Can you work these out from the model? Positions are in its coordinate system, mm. Face numbers are marked on the shaded views. A direction names the side the tool comes from. Give positions to 0.01 mm unless a question says otherwise; leave off trailing zeros. Order: outer loops, then holes, each group sorted by start corner. A loop starts at its lowest first (then second) coordinate and runs counter-clockwise, first axis right, second up. Notation, with made-up numbers: M -38.75,-9.75 L -21.75,-9.75 A32 cw -21.75,26.25 Z; hole C 76.25,0.25 d1. An arc over 180 degrees is marked long. Answer as a JSON object with one key per item and string values.
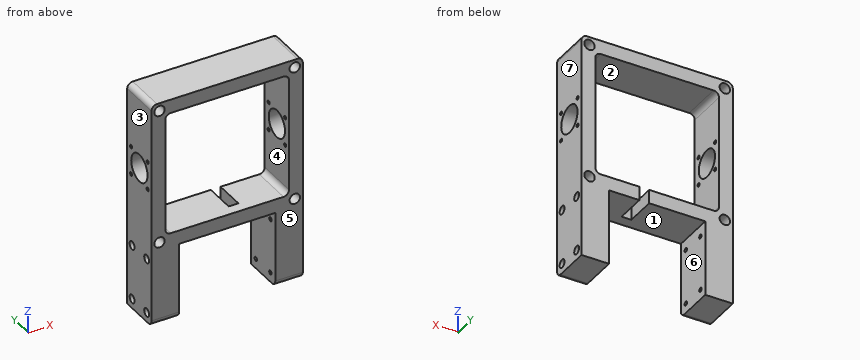
```python
from build123d import *

# Parameters (mm, degrees)
SKETCH1_W           = 25.4
SKETCH1_H           = 69.85
SKETCH1_R           = 4.826
SKETCH1_W_2         = 114.3
SKETCH1_H_2         = 114.3
BOSS_EXTRUDE2_DEPTH = 38.1
CUT_EXTRUDE1_REACH  = 203.206
SKETCH5_R           = 1.63195
SKETCH5_R_2         = 12.75
SKETCH7_W           = 12.7
SKETCH7_H           = 27.94
CUT_EXTRUDE2_DEPTH  = 4.5
CUT_EXTRUDE3_REACH  = 203.206
SKETCH10_R          = 1.905
SKETCH10_3_R        = 3.81
SKETCH10_3_R_2      = 1.905
CUT_EXTRUDE4_DEPTH  = 15.24
CUT_EXTRUDE5_START  = -15.24
SKETCH11_R          = 3.81
CUT_EXTRUDE5_DEPTH  = 15.24
FILLET10_R          = 5.08
FILLET11_R          = 5.08
FILLET12_R          = 5.08
FILLET13_R          = 5.08
FILLET14_R          = 5.08
FILLET15_R          = 5.08
FILLET16_R          = 5.08


with BuildPart() as part:
    # Sketch1 → Boss-Extrude2 (new body)
    # profile 1 of 3: a face of its own
    with BuildSketch(Plane(origin=(0, 0, 0), x_dir=(1, 0, 0), z_dir=(0, 1, 0))):
        with Locations((-57.15, 104.775)):
            Rectangle(SKETCH1_W, SKETCH1_H)
    # profile 2 of 3: a face of its own
    with BuildSketch(Plane(origin=(0, 0, 0), x_dir=(1, 0, 0), z_dir=(0, 1, 0))):
        Polygon((-44.45, 69.85), (-69.85, 69.85), (-69.85, -69.85), (69.85, -69.85), (69.85, 69.85), (44.45, 69.85), (-31.75, 69.85), align=None)
        with Locations(Location((-62.484, -62.484, 0), (0, 0, 90))):
            Circle(SKETCH1_R, mode=Mode.SUBTRACT)
        Rectangle(SKETCH1_W_2, SKETCH1_H_2, mode=Mode.SUBTRACT)
        with Locations(Location((62.484, -62.484, 0), (0, 0, 90))):
            Circle(SKETCH1_R, mode=Mode.SUBTRACT)
        with Locations(Location((-62.484, 62.484, 0), (0, 0, 90))):
            Circle(SKETCH1_R, mode=Mode.SUBTRACT)
        with Locations(Location((62.484, 62.484, 0), (0, 0, 90))):
            Circle(SKETCH1_R, mode=Mode.SUBTRACT)
    # profile 3 of 3: a face of its own
    with BuildSketch(Plane(origin=(0, 0, 0), x_dir=(1, 0, 0), z_dir=(0, 1, 0))):
        with Locations((57.15, 104.775)):
            Rectangle(SKETCH1_W, SKETCH1_H)
    extrude(amount=BOSS_EXTRUDE2_DEPTH)

    # Cut-Extrude1: up to this face of the body (flat: up to its plane)
    cut_extrude1_end = Plane(part.part.faces().sort_by_distance((-69.85, 19.05, -34.925))[0])
    # Sketch5 → Cut-Extrude1 (cut, up to the picked face)
    with BuildSketch(Plane(origin=(69.85, 0, 0), x_dir=(0, 0, -1), z_dir=(1, 0, 0)), mode=Mode.PRIVATE) as cut_extrude1_sk1:
        with Locations((-13, 32.05)):
            Circle(SKETCH5_R)
    cut_extrude1_tool1 = split(extrude(cut_extrude1_sk1.sketch, amount=-CUT_EXTRUDE1_REACH, mode=Mode.PRIVATE), bisect_by=cut_extrude1_end, keep=Keep.BOTH, mode=Mode.PRIVATE)
    # Sketch5 → Cut-Extrude1 (cut, up to the picked face)
    with BuildSketch(Plane(origin=(69.85, 0, 0), x_dir=(0, 0, -1), z_dir=(1, 0, 0)), mode=Mode.PRIVATE) as cut_extrude1_sk2:
        with Locations((13, 6.05)):
            Circle(SKETCH5_R)
    cut_extrude1_tool2 = split(extrude(cut_extrude1_sk2.sketch, amount=-CUT_EXTRUDE1_REACH, mode=Mode.PRIVATE), bisect_by=cut_extrude1_end, keep=Keep.BOTH, mode=Mode.PRIVATE)
    # Sketch5 → Cut-Extrude1 (cut, up to the picked face)
    with BuildSketch(Plane(origin=(69.85, 0, 0), x_dir=(0, 0, -1), z_dir=(1, 0, 0)), mode=Mode.PRIVATE) as cut_extrude1_sk3:
        with Locations((-13, 6.05)):
            Circle(SKETCH5_R)
    cut_extrude1_tool3 = split(extrude(cut_extrude1_sk3.sketch, amount=-CUT_EXTRUDE1_REACH, mode=Mode.PRIVATE), bisect_by=cut_extrude1_end, keep=Keep.BOTH, mode=Mode.PRIVATE)
    # Sketch5 → Cut-Extrude1 (cut, up to the picked face)
    with BuildSketch(Plane(origin=(69.85, 0, 0), x_dir=(0, 0, -1), z_dir=(1, 0, 0)), mode=Mode.PRIVATE) as cut_extrude1_sk4:
        with Locations((13, 32.05)):
            Circle(SKETCH5_R)
    cut_extrude1_tool4 = split(extrude(cut_extrude1_sk4.sketch, amount=-CUT_EXTRUDE1_REACH, mode=Mode.PRIVATE), bisect_by=cut_extrude1_end, keep=Keep.BOTH, mode=Mode.PRIVATE)
    # Sketch5 → Cut-Extrude1 (cut, up to the picked face)
    with BuildSketch(Plane(origin=(69.85, 0, 0), x_dir=(0, 0, -1), z_dir=(1, 0, 0)), mode=Mode.PRIVATE) as cut_extrude1_sk5:
        with Locations((0, 19.05)):
            Circle(SKETCH5_R_2)
    cut_extrude1_tool5 = split(extrude(cut_extrude1_sk5.sketch, amount=-CUT_EXTRUDE1_REACH, mode=Mode.PRIVATE), bisect_by=cut_extrude1_end, keep=Keep.BOTH, mode=Mode.PRIVATE)
    add(cut_extrude1_tool1.solids().sort_by(Axis((69.85, 32.05, 13), (-1, 0, 0)))[0], mode=Mode.SUBTRACT)
    add(cut_extrude1_tool2.solids().sort_by(Axis((69.85, 6.05, -13), (-1, 0, 0)))[0], mode=Mode.SUBTRACT)
    add(cut_extrude1_tool3.solids().sort_by(Axis((69.85, 6.05, 13), (-1, 0, 0)))[0], mode=Mode.SUBTRACT)
    add(cut_extrude1_tool4.solids().sort_by(Axis((69.85, 32.05, -13), (-1, 0, 0)))[0], mode=Mode.SUBTRACT)
    add(cut_extrude1_tool5.solids().sort_by(Axis((69.85, 19.05, 0), (-1, 0, 0)))[0], mode=Mode.SUBTRACT)

    # Sketch7 → Cut-Extrude2 (cut, symmetric)
    with BuildSketch(Plane.ZY.offset(-11.879999989)):
        with Locations((-63.5, 24.13)):
            Rectangle(SKETCH7_W, SKETCH7_H)
    extrude(amount=CUT_EXTRUDE2_DEPTH, both=True, mode=Mode.SUBTRACT)

    # Cut-Extrude3: up to this face of the body (flat: up to its plane)
    cut_extrude3_end = Plane(part.part.faces().sort_by_distance((-69.85, 19.05, -37.47957558))[0])
    # Sketch10 → Cut-Extrude3 (cut, up to the picked face)
    with BuildSketch(Plane(origin=(69.85, 0, 0), x_dir=(0, 0, -1), z_dir=(1, 0, 0)), mode=Mode.PRIVATE) as cut_extrude3_sk1:
        with Locations((80.01, 30.48)):
            Circle(SKETCH10_R)
    cut_extrude3_tool1 = split(extrude(cut_extrude3_sk1.sketch, amount=-CUT_EXTRUDE3_REACH, mode=Mode.PRIVATE), bisect_by=cut_extrude3_end, keep=Keep.BOTH, mode=Mode.PRIVATE)
    # Sketch10 → Cut-Extrude3 (cut, up to the picked face)
    with BuildSketch(Plane(origin=(69.85, 0, 0), x_dir=(0, 0, -1), z_dir=(1, 0, 0)), mode=Mode.PRIVATE) as cut_extrude3_sk2:
        with Locations((80.01, 7.62)):
            Circle(SKETCH10_R)
    cut_extrude3_tool2 = split(extrude(cut_extrude3_sk2.sketch, amount=-CUT_EXTRUDE3_REACH, mode=Mode.PRIVATE), bisect_by=cut_extrude3_end, keep=Keep.BOTH, mode=Mode.PRIVATE)
    # Sketch10 → Cut-Extrude3 (cut, up to the picked face)
    with BuildSketch(Plane(origin=(69.85, 0, 0), x_dir=(0, 0, -1), z_dir=(1, 0, 0)), mode=Mode.PRIVATE) as cut_extrude3_sk3:
        with Locations((130.81, 30.48)):
            Circle(SKETCH10_R)
    cut_extrude3_tool3 = split(extrude(cut_extrude3_sk3.sketch, amount=-CUT_EXTRUDE3_REACH, mode=Mode.PRIVATE), bisect_by=cut_extrude3_end, keep=Keep.BOTH, mode=Mode.PRIVATE)
    # Sketch10 → Cut-Extrude3 (cut, up to the picked face)
    with BuildSketch(Plane(origin=(69.85, 0, 0), x_dir=(0, 0, -1), z_dir=(1, 0, 0)), mode=Mode.PRIVATE) as cut_extrude3_sk4:
        with Locations((130.81, 7.62)):
            Circle(SKETCH10_R)
    cut_extrude3_tool4 = split(extrude(cut_extrude3_sk4.sketch, amount=-CUT_EXTRUDE3_REACH, mode=Mode.PRIVATE), bisect_by=cut_extrude3_end, keep=Keep.BOTH, mode=Mode.PRIVATE)
    add(cut_extrude3_tool1.solids().sort_by(Axis((69.85, 30.48, -80.01), (-1, 0, 0)))[0], mode=Mode.SUBTRACT)
    add(cut_extrude3_tool2.solids().sort_by(Axis((69.85, 7.62, -80.01), (-1, 0, 0)))[0], mode=Mode.SUBTRACT)
    add(cut_extrude3_tool3.solids().sort_by(Axis((69.85, 30.48, -130.81), (-1, 0, 0)))[0], mode=Mode.SUBTRACT)
    add(cut_extrude3_tool4.solids().sort_by(Axis((69.85, 7.62, -130.81), (-1, 0, 0)))[0], mode=Mode.SUBTRACT)

    # Sketch10<3> → Cut-Extrude4 (cut)
    # profile 1 of 4: a face of its own
    with BuildSketch(Plane(origin=(69.85, 0, 0), x_dir=(0, 0, -1), z_dir=(1, 0, 0))):
        with Locations((80.01, 30.48)):
            Circle(SKETCH10_3_R)
        with Locations((80.01, 30.48)):
            Circle(SKETCH10_3_R_2, mode=Mode.SUBTRACT)
    # profile 2 of 4: a face of its own
    with BuildSketch(Plane(origin=(69.85, 0, 0), x_dir=(0, 0, -1), z_dir=(1, 0, 0))):
        with Locations((130.81, 7.62)):
            Circle(SKETCH10_3_R)
        with Locations((130.81, 7.62)):
            Circle(SKETCH10_3_R_2, mode=Mode.SUBTRACT)
    # profile 3 of 4: a face of its own
    with BuildSketch(Plane(origin=(69.85, 0, 0), x_dir=(0, 0, -1), z_dir=(1, 0, 0))):
        with Locations((130.81, 30.48)):
            Circle(SKETCH10_3_R)
        with Locations((130.81, 30.48)):
            Circle(SKETCH10_3_R_2, mode=Mode.SUBTRACT)
    # profile 4 of 4: a face of its own
    with BuildSketch(Plane(origin=(69.85, 0, 0), x_dir=(0, 0, -1), z_dir=(1, 0, 0))):
        with Locations((80.01, 7.62)):
            Circle(SKETCH10_3_R)
        with Locations((80.01, 7.62)):
            Circle(SKETCH10_3_R_2, mode=Mode.SUBTRACT)
    extrude(amount=-CUT_EXTRUDE4_DEPTH, mode=Mode.SUBTRACT)

    # Sketch11 → Cut-Extrude5 (cut)
    with BuildSketch(Plane.ZY.offset(69.85).offset(CUT_EXTRUDE5_START)):
        with Locations(Location((-130.81, 30.48, 0), (0, 0, 180))):
            Circle(SKETCH11_R)
        with Locations(Location((-80.01, 7.62, 0), (0, 0, 180))):
            Circle(SKETCH11_R)
        with Locations(Location((-80.01, 30.48, 0), (0, 0, 180))):
            Circle(SKETCH11_R)
        with Locations(Location((-130.81, 7.62, 0), (0, 0, 180))):
            Circle(SKETCH11_R)
    extrude(amount=CUT_EXTRUDE5_DEPTH, mode=Mode.SUBTRACT)

    # Fillet10
    fillet10_edges = [part.edges().sort_by_distance(p)[0] for p in [
        (57.15, 19.05, -57.15),
    ]]
    fillet(fillet10_edges, radius=FILLET10_R)

    # Fillet11
    fillet11_edges = [part.edges().sort_by_distance(p)[0] for p in [
        (-57.15, 19.05, -57.15),
    ]]
    fillet(fillet11_edges, radius=FILLET11_R)

    # Fillet12
    fillet12_edges = [part.edges().sort_by_distance(p)[0] for p in [
        (-57.15, 19.05, 57.15),
    ]]
    fillet(fillet12_edges, radius=FILLET12_R)

    # Fillet13
    fillet13_edges = [part.edges().sort_by_distance(p)[0] for p in [
        (57.15, 19.05, 57.15),
    ]]
    fillet(fillet13_edges, radius=FILLET13_R)

    # Fillet14
    fillet14_edges = [part.edges().sort_by_distance(p)[0] for p in [
        (-57.15, 0, -139.7),
        (57.15, 0, -139.7),
    ]]
    fillet(fillet14_edges, radius=FILLET14_R)

    # Fillet15
    fillet15_edges = [part.edges().sort_by_distance(p)[0] for p in [
        (-69.85, 19.05, 69.85),
    ]]
    fillet(fillet15_edges, radius=FILLET15_R)

    # Fillet16
    fillet16_edges = [part.edges().sort_by_distance(p)[0] for p in [
        (69.85, 19.05, 69.85),
    ]]
    fillet(fillet16_edges, radius=FILLET16_R)


solid = part.part
```
1) I need wall thicknesses on L1, parallel to Y at x = -62, z = -80; L2, parallel to Y at x = -63.75, z = -13; L3, parallel to X at y = 5.5, z = -118.5. Which ranges of each line are inside material? Lowest first, please.
Results found:
{"L1": "y = 0 to 3.81, 11.43 to 26.67, 34.29 to 38.1", "L2": "y = 0 to 4.42, 7.68 to 30.42, 33.68 to 38.1", "L3": "x = -69.85 to -44.45, 44.45 to 69.85"}
2) I want a section at A-A on x = -22. Write out the boundary of the cut face in (y, z), and give its area (3 significant figures).
Results found:
{"outline": "M 0,-69.85 L 38.1,-69.85 L 38.1,-57.15 L 0,-57.15 Z; M 0,57.15 L 38.1,57.15 L 38.1,69.85 L 0,69.85 Z", "area": "968 mm²"}
3) For the marked faces 1, 2 and 3, which set-ups out of +Z, -Z, +X, -X, +Y, -Y let a thin tool reach every point of the face, with its end or its side?
Results found:
{"face 1": "-Z, +Y, -Y", "face 2": "+Y, -Y", "face 3": "+Z, -Z, -X, +Y, -Y"}
4) I want a section at B-B on y = 19.05. Count the separate pieces of the cut face and the enclosed holes in it, and give its area (3 significant figures).
Results found:
{"separate pieces": "3", "enclosed holes": "4", "area": "8,960 mm²"}
5) I want a section at C-C on z = 19.5. Write out the boundary of the cut face in (x, y).
Results found:
{"outline": "M -69.85,0 L -57.15,0 L -57.15,38.1 L -69.85,38.1 Z; M 57.15,0 L 69.85,0 L 69.85,38.1 L 57.15,38.1 Z"}
6) I'm going to push flat-ended pins straight in: pin 1 Ø11.5 at (x, y) = (-21, 15.5) entering from -Z; pin 2 Ø2.5 at (y, z) = (9, -78.5) entering from +X; pin 3 Ø3 at (y, z) = (30.48, -130.81) entering from -X. Where does each tip first touch, or does it pass through?
Results found:
{"pin 1": "stops at z = -69.85", "pin 2": "stops at x = 54.61", "pin 3": "passes through"}
7) Thinking about a two-plate mould opening in X: for the marked faces 4, 5, 6 and 7, which applies, pulls with the +X half, pulls with the -X half, needs draft (parallel to the pull), parting line crosses it, or undercut?
Results found:
{"face 4": "undercut", "face 5": "needs draft", "face 6": "undercut", "face 7": "pulls with the +X half"}
